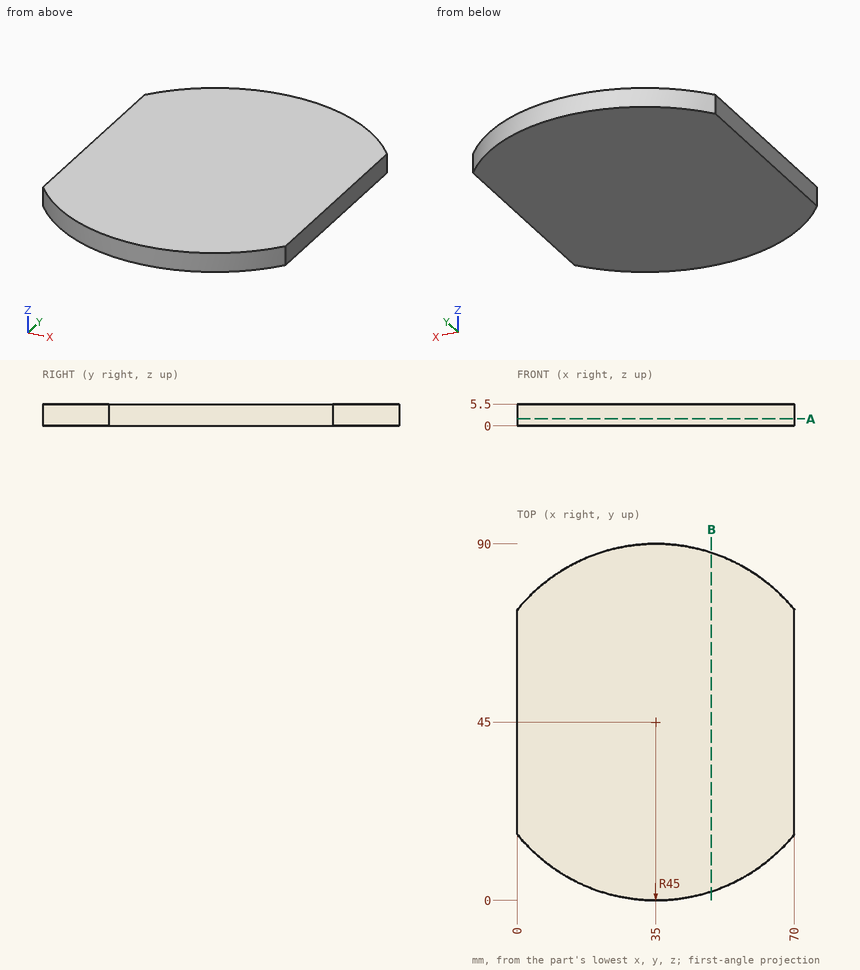
Geometry: see drawing. Coordinates: mm, zero at the bounding-box minimum. Give positions to 0.01 mm unless a question says otherwise; leave off trailing zeros. Loops run counter-clockwise (first coordinate to the right, second up) from the corner with the lowest first, then second, coordinate; pieces in that order, holes last. Notation, with made-up numbers: (73.5, 65.5) -> (84.5, 65.5) arc R18 ccw to (84.5, 83.5) -> close; hole circle Ø10 at (77, -1). An arc over 180 degrees is marked (long way). Use CSV: the item, a comma, the result in double quotes.
(1) Cut plane B-B (x = 49). Output: boundary loops of the cut face in (y, z), plus the area to 3 significant figures.
From the geometry:
outline,"(2.23, 0) -> (87.77, 0) -> (87.77, 5.5) -> (2.23, 5.5) -> close"
area,"470 mm^2"
(2) Cut plane A-A (z = 1.75). Output: boundary loops of the cut face in (x, y), plus the area to 3 significant figures.
From the geometry:
outline,"(0, 16.72) arc R45 ccw to (70, 16.72) -> (70, 73.28) arc R45 ccw to (0, 73.28) -> close"
area,"5,590 mm^2"
(3) Ray query, line 1 along X through (y, z) = (13.5, 1.7); line 2 along X through (y, z) = (13, 0.7); line 3 along Y through (x, z) = (62, 5). Return the intervals inside material, ascending. Write a range as [from, to].
From the geometry:
line 1,"[2.86, 67.14]"
line 2,"[3.36, 66.64]"
line 3,"[9, 81]"
